```python
from build123d import *

# Parameters (mm, degrees)
SKETCH1_R           = 39.75
BOSS_EXTRUDE1_DEPTH = 8
CHAMFER1_SIZE       = 1
SKETCH2_R           = 9
SKETCH2_R_2         = 4
BOSS_EXTRUDE2_DEPTH = 8
BOSS_EXTRUDE3_START = 8
SKETCH2_3_R         = 4
BOSS_EXTRUDE3_DEPTH = 7
FILLET1_R           = 63
CHAMFER2_SIZE       = 1


with BuildPart() as part:
    # Sketch1 → Boss-Extrude1 (new body)
    with BuildSketch(Plane.XY):
        Circle(SKETCH1_R)
    extrude(amount=BOSS_EXTRUDE1_DEPTH)

    # Chamfer1
    chamfer1_edges = [part.edges().sort_by_distance(p)[0] for p in [
        (-39.75, 0, 0),
    ]]
    chamfer(chamfer1_edges, length=CHAMFER1_SIZE)

    # Sketch2 → Boss-Extrude2 (add)
    # profile 1 of 2: a face of its own
    with BuildSketch(Plane.XY.offset(8)):
        Circle(SKETCH2_R)
        Circle(SKETCH2_R_2, mode=Mode.SUBTRACT)
    # profile 2 of 2: a face of its own
    with BuildSketch(Plane.XY.offset(8)):
        Circle(SKETCH2_R_2)
    extrude(amount=BOSS_EXTRUDE2_DEPTH)

    # Sketch2<3> → Boss-Extrude3 (add)
    with BuildSketch(Plane.XY.offset(8).offset(BOSS_EXTRUDE3_START)):
        Circle(SKETCH2_3_R)
    extrude(amount=BOSS_EXTRUDE3_DEPTH)

    # Fillet1
    # the kernel refuses this fillet: 63 mm, written as the material it adds along each edge
    with BuildSketch(Plane(origin=(0, 0, 8), x_dir=(1, 0, 0), z_dir=(0, -1, 0))) as fillet1_piece_1:
        with BuildLine():
            CenterArc((39.724582991, 63), FILLET1_R, 240.811017564, 29.188982436)
            Line((9, 8), (9, 0))
            Line((9, 0), (39.724582991, 0))
        make_face()
    revolve(axis=Axis((0, 0, 8), (0, 0, 1)))

    # Chamfer2
    chamfer2_edges = [part.edges().sort_by_distance(p)[0] for p in [
        (-4, 0, 23),
    ]]
    chamfer(chamfer2_edges, length=CHAMFER2_SIZE)


solid = part.part
```
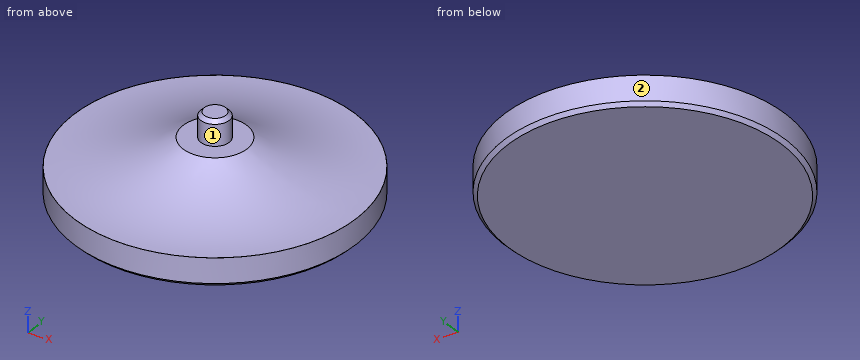
The model under review builds one solid part; all positions refer to its coordinate system, in mm. Face numbers are marked on the shaded views. A direction names the side the tool comes from. Coordinates: 2 decimals unless noted, no trailing zeros. Write each loop counter-clockwise with the first axis right and the second up, starting at its lowest first coordinate (ties: lowest second). Pieces come first, ordered by that corner, then holes. Notation, with made-up numbers: (13.25, 13) - (45.25, 13) arc R15 cw to (45.25, 36) - close; hole circle Ø7 at (-36.75, -19). An arc over 180 degrees is marked (long way). Write item = value, one per line.
(1) For line 1 (Z direction, x = 6, y = 1.5); line 2 (Y direction, x = -31, z = 6.5); line 3 (Y direction, x = -27, z = 5.25), list the stretches that pass through material, from the lowest coordinate up. Write a range as [from, to].
Result sheet:
line_1 = [0, 16]
line_2 = [-24.88, 24.88]
line_3 = [-29.17, 29.17]
(2) For P1, Ø2, axis at x = 17.5, z = 5, coming from the +Y side; P2, Ø6, axis at x = -27.5, y = 10.5, coming from the -Z side; P3, Ø5, axis at x = 25.5, z = 10, coming from the -Y side; P4, Ø8, axis at y = 4.5, z = 10, coming from the -X side, all flat-tipped, find the tip position at first contact; note any pin that passes through.
Result sheet:
P1 = 36.16
P2 = 0
P3 = -31.69
P4 = -39.74
(3) Machinability: for the marked faces 1 and 2, which of the approach directions +Z, -Z, +X, -X, +Y, -Y give a long, thin tool a straight path to every point of the face, cutting with its end or side? Answer none if there is none.
Result sheet:
face_1 = +Z
face_2 = +Z, -Z
(4) Consider section A-A, the plane z = 5.25. Give the boundary of the cut face in (x, y).
Result sheet:
outline = circle Ø79.5 at (0, 0)
